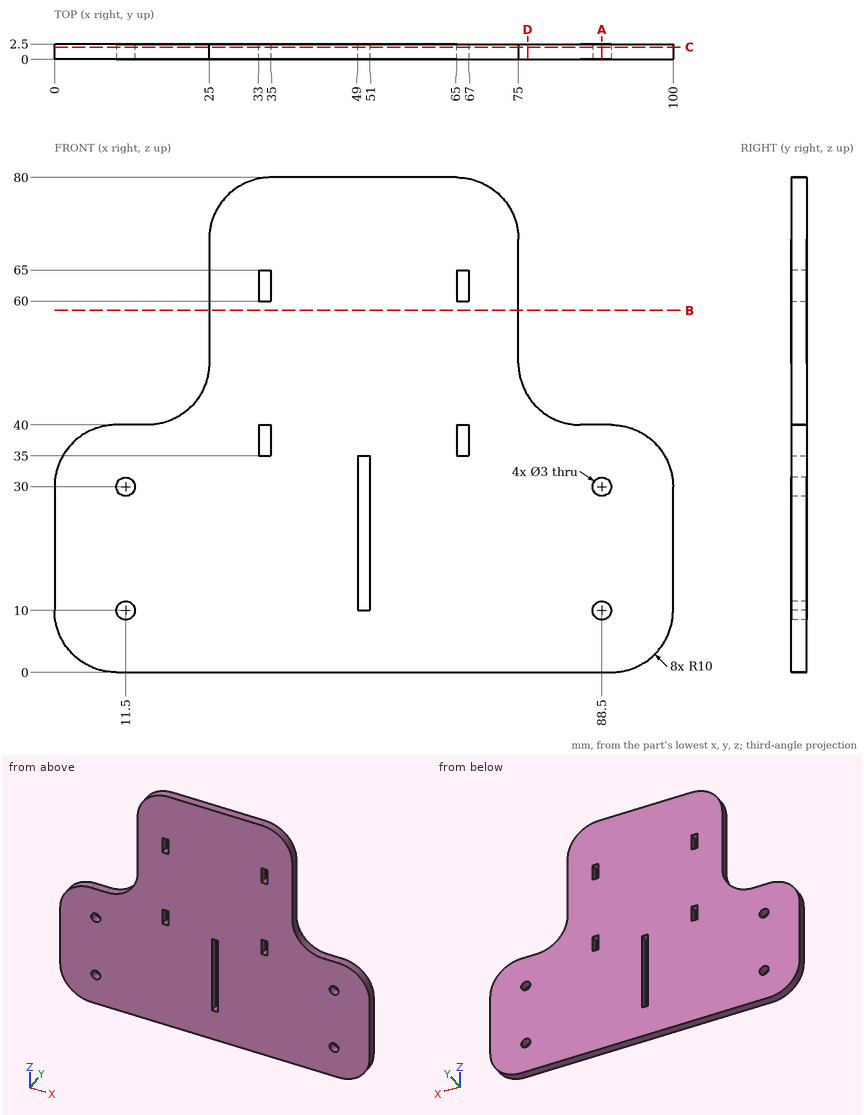
Geometry: see drawing. Coordinates: mm, zero at the bounding-box minimum. Give positions to 0.01 mm unless a question says otherwise; leave off trailing zeros. Loops run counter-clockwise (first coordinate to the right, second up) from the corner with the lowest first, then second, coordinate; pieces in that order, holes last. Notation, with made-up numbers: (-6, -21.5) -> (16, -21.5) arc R34 ccw to (16, 10.5) -> close; hole circle Ø3 at (10.5, -40). An arc over 180 degrees is marked (long way). Use one line per item in the form item = value.
Item 1: Section query D-D on x = 76.5. Output: boundary loops of the cut face in (y, z), and give its area (3 significant figures).
A:
outline = (0, 0) -> (2.5, 0) -> (2.5, 44.73) -> (0, 44.73) -> close
area = 112 mm^2
Item 2: Line query: probe 1 along X at (y, z) = (1, 30); probe 2 along Z at (x, y) = (88.5, 1.9); probe 3 along X at (y, z) = (1.55, 26). Output: solid intervals per line, ascending.
A:
probe_1 = 0 to 10, 13 to 49, 51 to 87, 90 to 100
probe_2 = 0 to 8.5, 11.5 to 28.5, 31.5 to 40
probe_3 = 0 to 49, 51 to 100
Item 3: Section query A-A on x = 88.5. Output: boundary loops of the cut face in (y, z).
A:
outline = (0, 0) -> (2.5, 0) -> (2.5, 8.5) -> (0, 8.5) -> close; (0, 11.5) -> (2.5, 11.5) -> (2.5, 28.5) -> (0, 28.5) -> close; (0, 31.5) -> (2.5, 31.5) -> (2.5, 40) -> (0, 40) -> close
Item 4: Section query B-B on z = 58.5. Output: boundary loops of the cut face in (x, y).
A:
outline = (25, 0) -> (75, 0) -> (75, 2.5) -> (25, 2.5) -> close
Item 5: Section query C-C on y = 2. Give the number of separate pieces and of enclosed holes in the cut face, and give its area (3 significant figures).
A:
separate_pieces = 1
enclosed_holes = 9
area = 5,800 mm^2
Item 6: Pin query (flat end, axial travel): P1, Ø0.8, axis at x = 11.5, y = 1, coming from the +Z side; P2, Ø1, axis at x = 34, y = 1, coming from the -Z side; P3, Ø1.2, axis at y = 1, z = 38, coming from the +X side; P4, Ø1.5, axis at y = 1, z = 32.5, coming from the +X side. Return the tip coordinate at first contact, or that it passes through.
A:
P1 = 40
P2 = 0
P3 = 96.73
P4 = 99.85
